Geometry: see drawing. Coordinates: mm, zero at the bounding-box minimum. A direction names the side the tool comes from. Coordinates: 2 decimals unless noted, no trailing zeros. Loops run counter-clockwise (first coordinate to the right, second up) from the corner with the lowest first, then second, coordinate; pieces in that order, holes last. Notation, with made-up numbers: (29.25, 83) - (75.25, 83) arc R21 cw to (75.25, 109) - close; hole circle Ø9 at (-0.75, 8). An arc over 180 degrees is marked (long way). Use one line per item in the form item = value.
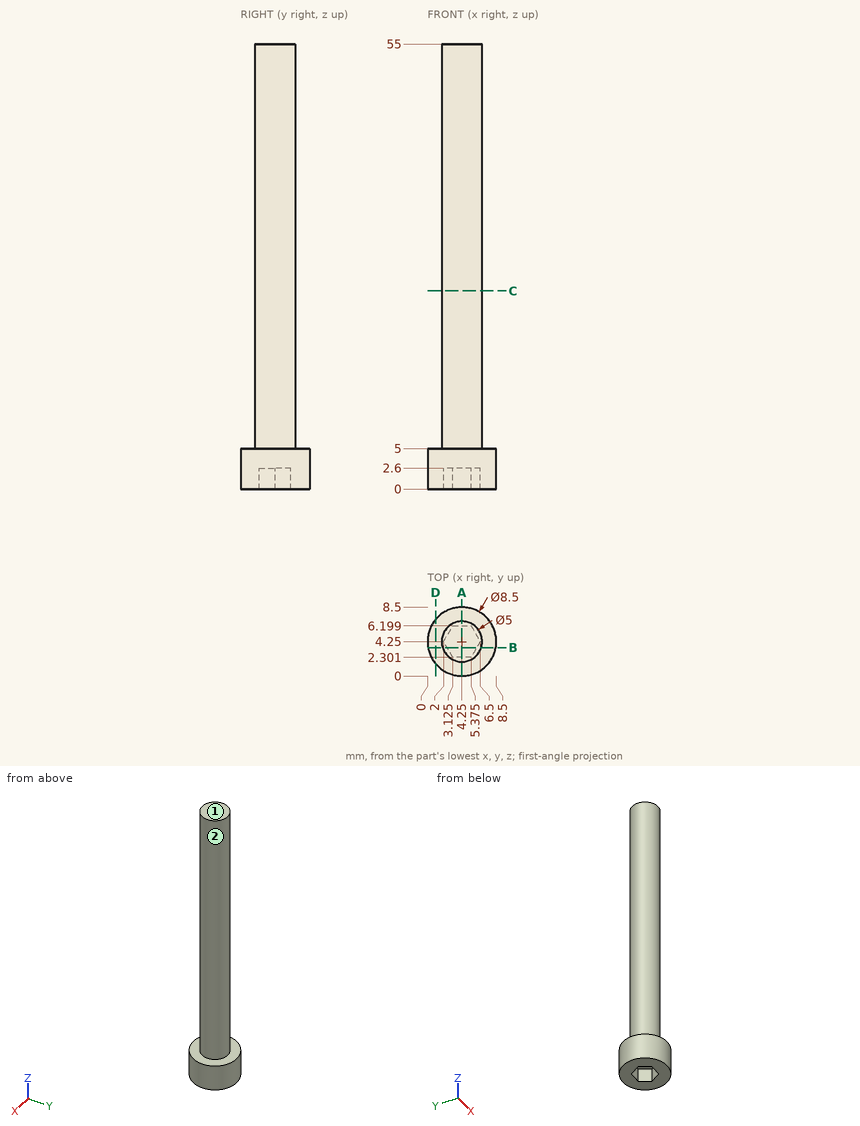
Q1. Cut plane C-C, the plane z = 24.5. Return loops of the section in (x, y), then the cut area to 3 significant figures.
Check values:
outline = circle Ø5 at (4.25, 4.25)
area = 19.6 mm²
Q2. Cut plane A-A, the plane x = 4.25. Return loops of the section in (y, z).
Check values:
outline = (0, 0) - (2.3, 0) - (2.3, 2.6) - (6.2, 2.6) - (6.2, 0) - (8.5, 0) - (8.5, 5) - (6.75, 5) - (6.75, 55) - (1.75, 55) - (1.75, 5) - (0, 5) - close
Q3. Cut plane B-B, the plane y = 3.5. Return loops of the section in (x, z) (1 decimal), then the cut area to 3 significant figures.
Check values:
outline = (0.1, 0) - (2.4, 0) - (2.4, 2.6) - (6.1, 2.6) - (6.1, 0) - (8.4, 0) - (8.4, 5) - (6.6, 5) - (6.6, 55) - (1.9, 55) - (1.9, 5) - (0.1, 5) - close
area = 271 mm²
Q4. Set-up query: the marked faces 1 and 2. Return all of +Z, -Z, +X, -X, +Y, -Y with unobstructed straight access to the full face (end or side cutting, diameter ignored); none if empty.
Check values:
face_1 = +Z, +X, -X, +Y, -Y
face_2 = +Z
Q5. Ray query, line 1 along Z through (x, y) = (4.25, 3.75); line 2 along Z through (x, y) = (3.25, 7); line 3 along Y through (x, z) = (6, 8) (1 decimal). Return the intervals inside material, ascending. Write a range as [from, to].
Check values:
line_1 = [2.6, 55]
line_2 = [0, 5]
line_3 = [2.5, 6]
Q6. Cut plane D-D, the plane x = 1. Return loops of the section in (y, z), then the cut area to 3 significant figures.
Check values:
outline = (1.51, 0) - (6.99, 0) - (6.99, 5) - (1.51, 5) - close
area = 27.4 mm²
Q7. First-contact query: P1, Ø0.7, axis at x = 3.5, z = 1, coming from the +Y side; P2, Ø3, axis at y = 4.5, z = 9, coming from the -X side; P3, Ø4, axis at y = 5, z = 21, coming from the +X side. Flat tips, straight axial feed; report the tip coordinate or a pass-through.
Check values:
P1 = 8.48
P2 = 1.75
P3 = 6.75
